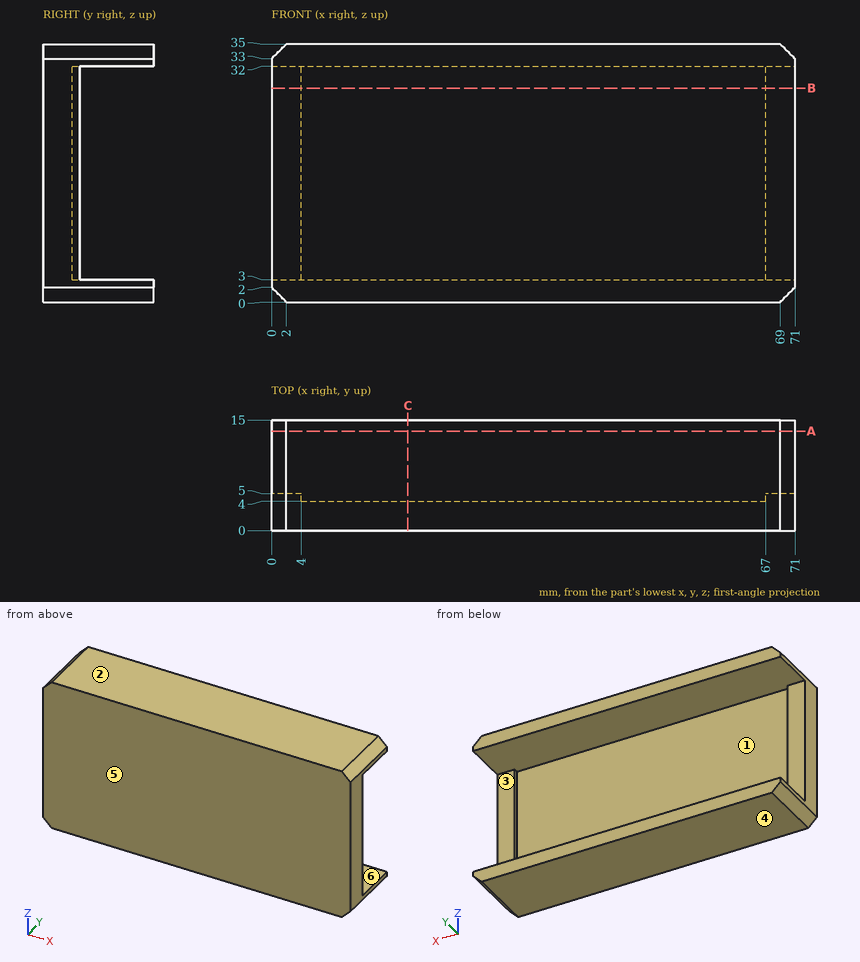
Geometry: see drawing. Coordinates: mm, zero at the bounding-box minimum. A direction names the side the tool comes from. Give positions to 0.01 mm unless a question says otherwise; leave off trailing zeros. Order: outer loops, then holes, each group sorted by start corner. A loop starts at its lowest first (then second) coordinate and runs counter-clockwise, first axis right, second up. Notation, with made-up numbers: (87.25, 85) -> (115.25, 85) arc R16 ccw to (115.25, 89) -> close; hole circle Ø9 at (-33, 49). An arc over 180 degrees is marked (long way). Write each question's results on one line, items separated by ' | '. Start each with the question number.
1) Set-up query: the marked faces 1, 2 and 3. Return all of +Z, -Z, +X, -X, +Y, -Y with unobstructed straight access to the full face (end or side cutting, diameter ignored); none if empty.
2) Draft query along Z for the marked faces 4, 5 and 6. Return one class per face: pulls with the +Z half, pulls with the -Z half, needs draft (parallel to the pull), parting line crosses it, or undercut.
3) Section C-C (x = 18.5). Return loops of the section in (y, z), then the cut area to 3 significant figures.
4) Section A-A (y = 13.5). Return loops of the section in (x, z), then the cut area to 3 significant figures.
5) Line query: line 1 (Z direction, x = 33.5, y = 12); line 2 (X direction, y = 4.75, z = 25.5); line 3 (Y direction, x = 59, z = 6.5). Output: solid intervals per line, ascending. Write a range as from..to.
6) First-contact query: pin 1 (12 mm diameter, centred on x = 57, z = 15.5, fed in from -Y); pin 2 (1 mm diameter, centred on x = 44, z = 12, fed in from +Y); pin 3 (3 mm diameter, centred on x = 1, z = 11, fed in from +Y). Flat tips, straight axial feed; report the tip coordinate or a pass-through.
7) Section B-B (z = 29). Return loops of the section in (x, y).
Calculated:
1) face 1: +Y | face 2: +Z, +X, -X, +Y, -Y | face 3: +X, -X, +Y
2) face 4: pulls with the -Z half | face 5: needs draft | face 6: undercut
3) outline: (0, 0) -> (15, 0) -> (15, 3) -> (4, 3) -> (4, 32) -> (15, 32) -> (15, 35) -> (0, 35) -> close | area: 206 mm2
4) outline: (0, 2) -> (2, 0) -> (69, 0) -> (71, 2) -> (71, 3) -> (0, 3) -> close; (0, 32) -> (71, 32) -> (71, 33) -> (69, 35) -> (2, 35) -> (0, 33) -> close | area: 418 mm2
5) line 1: 0..3, 32..35 | line 2: 0..4, 67..71 | line 3: 0..4
6) pin 1: y = 0 | pin 2: y = 4 | pin 3: y = 5
7) outline: (0, 0) -> (71, 0) -> (71, 5) -> (67, 5) -> (67, 4) -> (4, 4) -> (4, 5) -> (0, 5) -> close
